Build history of the part. All positions in model axes, mm. Face numbers are marked on the shaded views. Coordinates: 2 decimals unless noted, no trailing zeros. Order: outer loops, then holes, each group sorted by start corner. A loop starts at its lowest first (then second) coordinate and runs counter-clockwise, first axis right, second up. Notation, with made-up numbers: (46.25, 21) - (74.25, 21) arc R23 ccw to (74.25, 54) - close; hole circle Ø7 at (11.5, 39). An arc over 180 degrees is marked (long way). Return JSON: item names as keys, results as strings.
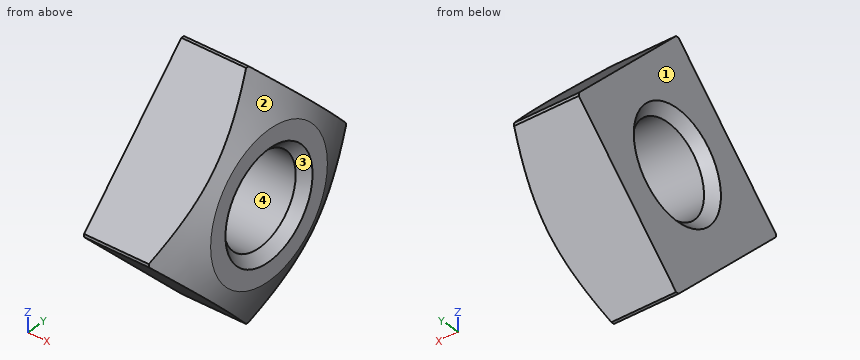
from build123d import *

# Parameters (mm, degrees)
SKETCH2_W          = 32
SKETCH2_H          = 32
CUT_EXTRUDE1_DEPTH = 4


with BuildPart() as part:
    # Sketch1 → Revolve1 (revolve)
    with BuildSketch(Plane.XY):
        Polygon((0, 0), (0, 5.656854249), (2.996951225, 5.656854249), (4, 3.35), (4, 0), align=None)
    revolve(axis=Axis((4, 0, 0), (-1, 0, 0)))

    # Sketch2 → Cut-Extrude1 (cut)
    with BuildSketch(Plane(origin=(0, 0, 0), x_dir=(0, 0, -1), z_dir=(1, 0, 0))):
        Rectangle(SKETCH2_W, SKETCH2_H)
        Polygon((-5.727564928, 0), (0, -5.727564928), (5.727564928, 0), (0, 5.727564928), align=None, mode=Mode.SUBTRACT)
    extrude(amount=CUT_EXTRUDE1_DEPTH, mode=Mode.SUBTRACT)

    # Sketch3 → Cut-Revolve1 (revolve, cut)
    with BuildSketch(Plane.XY):
        Polygon((0, 0), (0, 2.5), (0.433, 2.067), (3.567, 2.067), (4, 2.5), (4, 0), align=None)
    revolve(axis=Axis((4, 0, 0), (-1, 0, 0)), mode=Mode.SUBTRACT)


solid = part.part
1. Probe L1, parallel to Z at x = 1.8, y = 0; L2, parallel to Z at x = 1, y = -1.5. List the from-to ranges inside material, lowest first.
Check values:
{"L1": "-5.66 to -2.07, 2.07 to 5.66", "L2": "-4.23 to -1.42, 1.42 to 4.23"}
2. Cut at B-B on x = 3.3. Give the cut face in (y, z).
Check values:
{"outline": "(-4.89, -0.84) - (-0.84, -4.89) arc R4.96 ccw to (0.84, -4.89) - (4.89, -0.84) arc R4.96 ccw to (4.89, 0.84) - (0.84, 4.89) arc R4.96 ccw to (-0.84, 4.89) - (-4.89, 0.84) arc R4.96 ccw to start; hole circle Ø4.13 at (0, 0)"}
3. Mould opens along Z. For the marked faces 1, 2, 3 and 4 say: pulls with the +Z half, pulls with the -Z half, needs draft (parallel to the pull), parting line crosses it, or undercut.
Check values:
{"face 1": "needs draft", "face 2": "parting line crosses it", "face 3": "undercut", "face 4": "undercut"}
4. Cut at A-A on x = 0.6. Give the cut face in (y, z).
Check values:
{"outline": "(-5.66, -0.07) - (-0.07, -5.66) arc R5.66 ccw to (0.07, -5.66) - (5.66, -0.07) arc R5.66 ccw to (5.66, 0.07) - (0.07, 5.66) arc R5.66 ccw to (-0.07, 5.66) - (-5.66, 0.07) arc R5.66 ccw to start; hole circle Ø4.13 at (0, 0)"}
5. Drop flat-ended pins along their axis: pin 1 (1.5 mm diameter, centred on x = 2, y = -3, fed in from -Z); pin 2 (2 mm diameter, centred on x = 0.5, y = -2, fed in from +Z). Give the stop position or say it passes through.
Check values:
{"pin 1": "z = -3.48", "pin 2": "z = 4.73"}
